```python
from build123d import *

# Parameters (mm, degrees)
SKETCH1_R                = 50.8
SKETCH1_R_2              = 38.9128
EXTRUDE1_DEPTH           = 12.7
CHAMFER1_SIZE            = 0.480314
CHAMFER2_SIZE            = 1.1557
CUT_EXTRUDE1_DEPTH       = 13.7
FILLET1_R                = 0.4064
CIRPATTERN1_COUNT        = 4
FILLET1_OF_CIRPATTERN1_R = 0.4064


with BuildPart() as part:
    # Sketch1 → Extrude1 (new body)
    with BuildSketch(Plane.XY):
        Circle(SKETCH1_R)
        Circle(SKETCH1_R_2, mode=Mode.SUBTRACT)
    extrude(amount=EXTRUDE1_DEPTH)

    # Chamfer1
    chamfer1_edges = [part.edges().sort_by_distance(p)[0] for p in [
        (-50.8, 0, 0),
        (-50.8, 0, 12.7),
    ]]
    chamfer(chamfer1_edges, length=CHAMFER1_SIZE)

    # Chamfer2
    chamfer2_edges = [part.edges().sort_by_distance(p)[0] for p in [
        (-38.9128, 0, 0),
        (-38.9128, 0, 12.7),
    ]]
    chamfer(chamfer2_edges, length=CHAMFER2_SIZE)

    # Sketch2 → Cut-Extrude1 (cut, through all)
    with BuildSketch(Plane.XY.offset(12.7)):
        with BuildLine():
            Line((33.605733555, 38.095861616), (31.808067181, 36.298195241))
            Line((31.808067181, 36.298195241), (36.298195241, 31.808067181))
            Line((36.298195241, 31.808067181), (38.095861616, 33.605733555))
            ThreePointArc((38.095861616, 33.605733555), (35.921024484, 35.921024484), (33.605733555, 38.095861616))
        make_face()
    cut_extrude1 = extrude(amount=-CUT_EXTRUDE1_DEPTH, mode=Mode.SUBTRACT)

    # Fillet1
    fillet1_edges = [part.edges().sort_by_distance(p)[0] for p in [
        (36.298195241, 31.808067181, 6.35),
        (31.808067181, 36.298195241, 6.35),
    ]]
    fillet(fillet1_edges, radius=FILLET1_R)

    # CirPattern1: Cut-Extrude1 ×4 about axis
    cirpattern1_axis = Axis((0, 0, 0), (0, 0, 1))
    for i in range(1, CIRPATTERN1_COUNT):
        add(cut_extrude1.rotate(cirpattern1_axis, i * 360 / CIRPATTERN1_COUNT), mode=Mode.SUBTRACT)

    # Fillet1 of CirPattern1
    fillet1_of_cirpattern1_edges = [part.edges().sort_by_distance(p)[0] for p in [
        (-31.808067181, 36.298195241, 6.35),
        (-36.298195241, 31.808067181, 6.35),
        (-36.298195241, -31.808067181, 6.35),
        (-31.808067181, -36.298195241, 6.35),
        (31.808067181, -36.298195241, 6.35),
        (36.298195241, -31.808067181, 6.35),
    ]]
    fillet(fillet1_of_cirpattern1_edges, radius=FILLET1_OF_CIRPATTERN1_R)


solid = part.part
```
Input: part model. Units: mm. Frame: model coordinates. A direction names the side the tool comes from. Give positions to 0.01 mm unless a question says otherwise; leave off trailing zeros. Order: outer loops, then holes, each group sorted by start corner. A loop starts at its lowest first (then second) coordinate and runs counter-clockwise, first axis right, second up. Notation, with made-up numbers: M -36.75,12 L -19.75,12 A30 ccw -19.75,38 Z; hole C -8,50.5 d8. An arc over 180 degrees is marked long. Return JSON: item names as keys, results as strings.
1) Access query for faces 5 (the face through (50.447, -0.511, 0.13)), 6 (the face through (34.081, -34.026, 6.439)). Directions: +Z, -Z, +X, -X, +Y, -Y. A direction counts if a zero-diameter tool reaches every point of the face in a straight line with its end or side. Return the directions, or none.
Taken from the geometry:
{"face 5": "-Z, +X", "face 6": "+Z, -Z"}
2) Section query C-C on z = 5. Output: boundary loops of the cut face in (x, y), and give its area (3 significant figures).
Taken from the geometry:
{"outline": "M -38.1,-33.61 L -36.59,-32.1 A0.41 cw -36.01,-32.1 L -32.1,-36.01 A0.41 cw -32.1,-36.59 L -33.61,-38.1 A50.8 ccw 33.61,-38.1 L 32.1,-36.59 A0.41 cw 32.1,-36.01 L 36.01,-32.1 A0.41 cw 36.59,-32.1 L 38.1,-33.61 A50.8 ccw 38.1,33.61 L 36.59,32.1 A0.41 cw 36.01,32.1 L 32.1,36.01 A0.41 cw 32.1,36.59 L 33.61,38.1 A50.8 ccw -33.61,38.1 L -32.1,36.59 A0.41 cw -32.1,36.01 L -36.01,32.1 A0.41 cw -36.59,32.1 L -38.1,33.61 A50.8 ccw Z; hole C 0,0 d77.83", "area": "3,280 mm2"}
3) Line query: L1, parallel to Y at x = 0, z = 9.25; L2, parallel to X at y = 9, z = 4; L3, parallel to X at y = 19, z = 3. Output: solid intervals per line, ascending. Write a range as [from, to].
Taken from the geometry:
{"L1": "y = [-50.8, -38.91], [38.91, 50.8]", "L2": "x = [-50, -37.86], [37.86, 50]", "L3": "x = [-47.11, -33.96], [33.96, 47.11]"}
4) Contact query for flat-ended pins moving along their axis: pin 1 (4 mm diameter, centred on x = 4.5, z = 6, fed in from +Y); pin 2 (1 mm diameter, centred on y = -10, z = 1.5, fed in from -X); pin 3 (4 mm diameter, centred on y = 18.5, z = 4.5, fed in from +X). Output: stop coordinate, or through.
Taken from the geometry:
{"pin 1": "stops at y = 50.74", "pin 2": "stops at x = -49.9", "pin 3": "stops at x = 48.05"}
5) Mould query, pull axis Y, two halves, no side actions, for faces 1 (the face through (0.511, 50.447, 0.13)), 2 (the face through (-34.026, -34.081, 6.439)), 3 (the face through (-34.081, 34.026, 6.439)), 4 (the face through (50.447, -0.511, 12.57)). Classes: released by +Y, released by -Y, zero draft, split by the parting line, or undercut.
Taken from the geometry:
{"face 1": "released by +Y", "face 2": "undercut", "face 3": "undercut", "face 4": "split by the parting line"}
6) Section query A-A on x = 0. Output: boundary loops of the cut face in (y, z).
Taken from the geometry:
{"outline": "M -50.8,0.48 L -50.32,0 L -40.07,0 L -38.91,1.16 L -38.91,11.54 L -40.07,12.7 L -50.32,12.7 L -50.8,12.22 Z; M 38.91,1.16 L 40.07,0 L 50.32,0 L 50.8,0.48 L 50.8,12.22 L 50.32,12.7 L 40.07,12.7 L 38.91,11.54 Z"}
